Autodesk Fusion 360 part; units mm, degrees
sketch "Skizze1" plane through (0, 0, 0) normal (0, 0, 1) x (1, 0, 0)
  line L0 (0, 10) -> (40, 10)
  line L1 (40, 10) -> (40, -20)
  line L2 (40, -20) -> (0, -20)
  line L3 (0, -20) -> (0, 10)
  dimension "d1" = 40
  dimension "d2" = 30
extrude "Extrusion1" add sketch "Skizze1" along normal blind 3
fillet "Abrundung1" radius 3 4 edges at (0, -20, 1.5) (40, -20, 1.5) (40, 10, 1.5) (0, 10, 1.5)
sketch "Skizze2" plane through (0, 0, 3) normal (0, 0, 1) x (-1, 0, 0)
  arc A0 (-3, -10) -> (0, -7) centre (-3, -7) ccw
  line L0 (0, -7) -> (0, 17)
  arc A1 (0, 17) -> (-3, 20) centre (-3, 17) ccw
  line L1 (-3, 20) -> (-37, 20)
  arc A2 (-37, 20) -> (-40, 17) centre (-37, 17) ccw
  line L2 (-40, 17) -> (-40, -7)
  arc A3 (-40, -7) -> (-37, -10) centre (-37, -7) ccw
  line L3 (-37, -10) -> (-3, -10)
  circle A4 centre (-30, 5) radius 5
extrude "Extrusion2" add sketch "Skizze2" along normal blind 40 contours A4
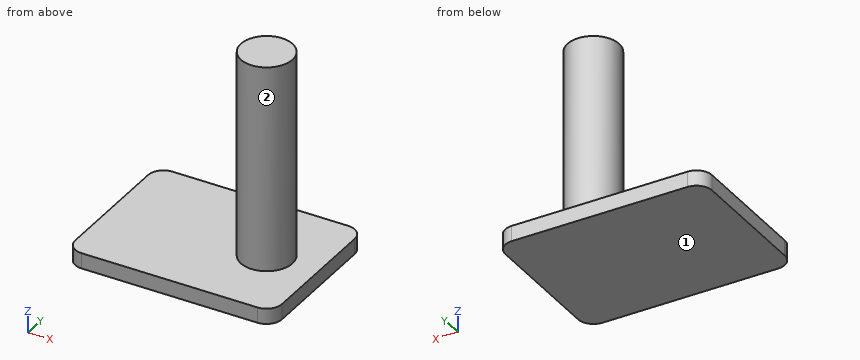
Could you check a few things on this model? Use its own coordinates, in mm. Face numbers are marked on the shaded views. A direction names the side the tool comes from. Give positions to 0.01 mm unless a question says otherwise; leave off trailing zeros. Loops run counter-clockwise (first coordinate to the right, second up) from the corner with the lowest first, then second, coordinate; pieces in that order, holes last. Notation, with made-up numbers: M 5.5,17.25 L 19.5,17.25 A11 ccw 19.5,34.25 Z; hole C 29.25,80 d3. An arc over 180 degrees is marked long. Answer as a JSON object with one key per item and string values.
Q1. Suppose I cut it at B-B, the plane y = -5. List the corners of the cut face in (x, z) for me, plus the area to 3 significant figures.
Values found:
{"outline": "M 0,0 L 40,0 L 40,3 L 35,3 L 35,43 L 25,43 L 25,3 L 0,3 Z", "area": "520 mm²"}
Q2. If I drill on probe 1 along Z at (x, y) = (13.5, -8.5); probe 2 along Y at (x, z) = (30, 40.5); probe 3 along Y at (x, z) = (32, 14), over which ranges is the centre line in solid material (lowest first)? Write a range as [from, to].
Values found:
{"probe 1": "z = [0, 3]", "probe 2": "y = [-10, 0]", "probe 3": "y = [-9.58, -0.42]"}
Q3. For P1, Ø10, axis at x = 30, z = 12.5, coming from the -Y side; P2, Ø15, axis at x = 10, y = -3.5, coming from the +Z side; P3, Ø1, axis at x = 27.5, z = 5.5, coming from the +Y side, each with a flat end and sliding along its axis, tell me the tip position at first contact or that it passes through.
Values found:
{"P1": "stops at y = -10", "P2": "stops at z = 3", "P3": "stops at y = -0.42"}
Q4. Suppose I cut it at A-A, the plane x = 33. List the corners of the cut face in (y, z) for me, plus the area to 3 significant figures.
Values found:
{"outline": "M -20,0 L 10,0 L 10,3 L -1,3 L -1,43 L -9,43 L -9,3 L -20,3 Z", "area": "410 mm²"}
Q5. Suppose I cut it at D-D, the plane y = -11.5. List the corners of the cut face in (x, z) for me, plus the area to 3 significant figures.
Values found:
{"outline": "M 0,0 L 40,0 L 40,3 L 0,3 Z", "area": "120 mm²"}
Q6. For the marked faces 1 and 2, which set-ups out of +Z, -Z, +X, -X, +Y, -Y let a thin tool reach every point of the face, with its end or its side?
Values found:
{"face 1": "-Z, +X, -X, +Y, -Y", "face 2": "+Z"}
Q7. Suppose I cut it at C-C, the plane z = 4. List the corners of the cut face in (x, y) for me.
Values found:
{"outline": "C 30,-5 d10"}
